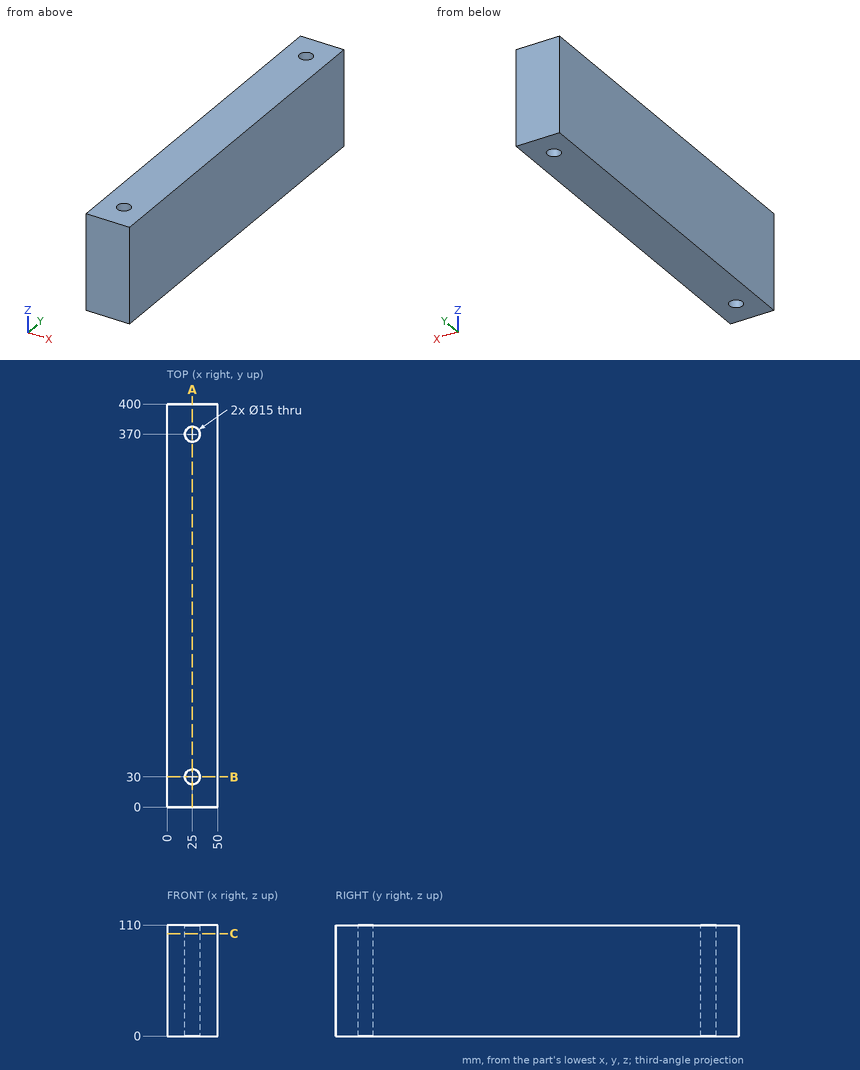
Geometry check sheet. Reference: drawing and pictorial views, mm from the part's lowest x, y, z. Coordinates: 2 decimals unless noted, no trailing zeros. Order: outer loops, then holes, each group sorted by start corner. A loop starts at its lowest first (then second) coordinate and runs counter-clockwise, first axis right, second up.
Item 1: Section check A-A (x = 25). Enter the section's corners in (y, z), plus the area to 3 significant figures.
Item 2: Section check C-C (z = 101.5). Enter the section's corners in (x, y), plus the area to 3 significant figures.
Item 3: Scan lines: line 1 along Y through (x, z) = (25, 35); line 2 along X through (y, z) = (30, 28); line 3 along Y through (x, z) = (27.5, 6). Record each from-to range of solid material in increasing order.
Item 4: Section check B-B (y = 30). Enter the section's corners in (x, z).
Check sheet entries:
1. outline: (0, 0) - (22.5, 0) - (22.5, 110) - (0, 110) - close; (37.5, 0) - (362.5, 0) - (362.5, 110) - (37.5, 110) - close; (377.5, 0) - (400, 0) - (400, 110) - (377.5, 110) - close
1. area: 40,700 mm2
2. outline: (0, 0) - (50, 0) - (50, 400) - (0, 400) - close; hole circle Ø15 at (25, 30); hole circle Ø15 at (25, 370)
2. area: 19,600 mm2
3. line 1: y = 0 to 22.5, 37.5 to 362.5, 377.5 to 400
3. line 2: x = 0 to 17.5, 32.5 to 50
3. line 3: y = 0 to 22.93, 37.07 to 362.93, 377.07 to 400
4. outline: (0, 0) - (17.5, 0) - (17.5, 110) - (0, 110) - close; (32.5, 0) - (50, 0) - (50, 110) - (32.5, 110) - close
